```python
from build123d import *

# Parameters (mm, degrees)
F1_DEPTH = 30
F2_DEPTH = 10
F3_R     = 5
F4_DEPTH = 20.8588644763


with BuildPart() as f1:
    # F0 (on Front) → F1 (new body, symmetric)
    with BuildSketch(Plane.XZ):
        with BuildLine():
            ThreePointArc((-10, 22.9128784748), (-18.5962121384, 16.7087071344), (-23.8484800354, 7.5))
            Line((-23.8484800354, 7.5), (-23.8484800354, -7.5))
            ThreePointArc((-23.8484800354, -7.5), (3.7939424821, -24.7104431454), (25, 0))
            ThreePointArc((25, 0), (20.9165006634, 13.6930639376), (10, 22.9128784748))
            Line((10, 22.9128784748), (10, 15))
            Line((10, 15), (0, 15))
            Line((0, 15), (-10, 15))
            Line((-10, 15), (-10, 22.9128784748))
        make_face()
        with BuildLine():
            ThreePointArc((15, 0), (-10.6066017178, -10.6066017178), (0, 15))
            ThreePointArc((0, 15), (10.6066017178, 10.6066017178), (15, 0))
        make_face(mode=Mode.SUBTRACT)
        with BuildLine():
            ThreePointArc((10, 22.9128784748), (0, 25), (-10, 22.9128784748))
            Line((-10, 22.9128784748), (-10, 15))
            Line((-10, 15), (0, 15))
            Line((0, 15), (10, 15))
            Line((10, 15), (10, 22.9128784748))
        make_face()
        with BuildLine():
            Line((-23.8484800354, -7.5), (-23.8484800354, 7.5))
            ThreePointArc((-23.8484800354, 7.5), (-25, 0), (-23.8484800354, -7.5))
        make_face()
        with BuildLine():
            Line((-10, 35), (-10, 22.9128784748))
            ThreePointArc((-10, 22.9128784748), (0, 25), (10, 22.9128784748))
            Line((10, 22.9128784748), (10, 35))
            Line((10, 35), (-10, 35))
        make_face()
    extrude(amount=F1_DEPTH, both=True)

    # F0 (on Front) → F2 (join, symmetric)
    with BuildSketch(Plane.XZ):
        with BuildLine():
            ThreePointArc((-23.8484800354, -7.5), (-25, 0), (-23.8484800354, 7.5))
            Line((-23.8484800354, 7.5), (-33.8484800354, 7.5))
            ThreePointArc((-33.8484800354, 7.5), (-38.8484800354, 2.5), (-43.8484800354, 7.5))
            Line((-43.8484800354, 7.5), (-98.8484800354, 7.5))
            ThreePointArc((-98.8484800354, 7.5), (-106.3484800354, 0), (-98.8484800354, -7.5))
            Line((-98.8484800354, -7.5), (-43.8484800354, -7.5))
            ThreePointArc((-43.8484800354, -7.5), (-38.8484800354, -2.5), (-33.8484800354, -7.5))
            Line((-33.8484800354, -7.5), (-23.8484800354, -7.5))
        make_face()
        with BuildLine():
            ThreePointArc((-98.8484800354, -4), (-102.8484800354, 0), (-98.8484800354, 4))
            Line((-98.8484800354, 4), (-78.8484800354, 4))
            ThreePointArc((-78.8484800354, 4), (-74.8484800354, 0), (-78.8484800354, -4))
            Line((-78.8484800354, -4), (-98.8484800354, -4))
        make_face(mode=Mode.SUBTRACT)
    extrude(amount=F2_DEPTH, both=True)

    # F3 (on face) → F4 (cut, through all)
    with BuildSketch(Plane.XY.offset(35)):
        with Locations((0, 15)):
            Circle(F3_R)
        with Locations((0, -15)):
            Circle(F3_R)
    extrude(amount=-F4_DEPTH, mode=Mode.SUBTRACT)


solid = f1.part
```
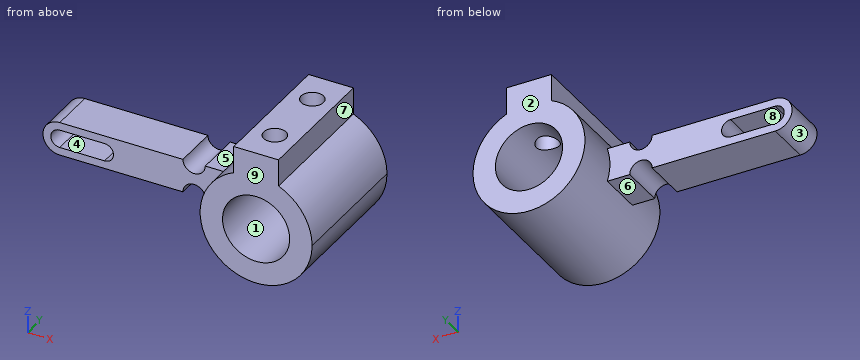
Geometry: final body of the model. Coordinates: model frame, mm. Face numbers are marked on the shaded views. A direction names the side the tool comes from. Coordinates: 2 decimals unless noted, no trailing zeros. Order: outer loops, then holes, each group sorted by start corner. A loop starts at its lowest first (then second) coordinate and runs counter-clockwise, first axis right, second up. Notation, with made-up numbers: (-10.5, 83) - (1.5, 83) arc R32 cw to (1.5, 110) - close; hole circle Ø1 at (7, 13.5). An arc over 180 degrees is marked (long way). Return JSON: item names as keys, results as strings. Group by question number.
1. Set-up query: the marked faces 5, 6, 7, 8 and 9. Return all of +Z, -Z, +X, -X, +Y, -Y with unobstructed straight access to the full face (end or side cutting, diameter ignored); none if empty.
2. Pin query (flat end, axial travel): pin 1 (4.5 mm diameter, centred on x = -54.5, z = -3, fed in from +Y); pin 2 (11 mm diameter, centred on x = -30, y = 4.5, fed in from -Z); pin 3 (6 mm diameter, centred on y = 14.5, z = 31.5, fed in from +X). Return the tip coordinate at first contact, or that it passes through.
3. Material intervals for line 1 along Y through (x, z) = (0, 27.25); line 2 along X through (y, z) = (3.5, 0); line 3 along X through (y, z) = (15, 26.75), sorted ascending. Write a range as [from, to].
4. Cut plane B-B (x = -91). Output: boundary loops of the cut face in (y, z).
5. Pull-direction query (Z, two-part tool) for the marked faces 1, 2, 3 and 4; classes: pulls with the +Z half, pulls with the -Z half, needs draft (parallel to the pull), parting line crosses it, or undercut.
6. Cut plane C-C (x = -67). Output: boundary loops of the cut face in (y, z).
Resolved:
{
 "1": {"face 5": "+Z, -X, +Y, -Y", "face 6": "-Z, -X, +Y, -Y", "face 7": "+Z, +X, +Y, -Y", "face 8": "+Y, -Y", "face 9": "+Z, -Z, +X, -X, -Y"},
 "2": {"pin 1": "stops at y = 10", "pin 2": "stops at z = -7.5", "pin 3": "stops at x = 10"},
 "3": {"line 1": "y = [-30, -20], [-10, 10], [20, 30]", "line 2": "x = [-106.35, -102.85], [-74.85, -15], [15, 25]", "line 3": "x = [-10, -5], [5, 10]"},
 "4": {"outline": "(-10, -7.5) - (10, -7.5) - (10, -4) - (-10, -4) - close; (-10, 4) - (10, 4) - (10, 7.5) - (-10, 7.5) - close"},
 "5": {"face 1": "undercut", "face 2": "needs draft", "face 3": "parting line crosses it", "face 4": "undercut"},
 "6": {"outline": "(-10, -7.5) - (10, -7.5) - (10, 7.5) - (-10, 7.5) - close"}
}
